```python
from build123d import *

# Parameters (mm, degrees)
SKIZZE1_R                       = 4.57
AUFSATZ_LINEAR_AUSTRAGEN1_DEPTH = 19
SCHNITT_LINEAR_AUSTRAGEN1_DEPTH = 20
VERRUNDUNG1_R                   = 0.5
KREISMUSTER1_COUNT              = 10
VERRUNDUNG1_OF_KREISMUSTER1_R   = 0.5
FASE1_SIZE                      = 0.2


with BuildPart() as part:
    # Skizze1 → Aufsatz-Linear austragen1 (new body)
    with BuildSketch(Plane(origin=(0, 0, 0), x_dir=(1, 0, 0), z_dir=(0, 1, 0))):
        Circle(SKIZZE1_R)
    extrude(amount=AUFSATZ_LINEAR_AUSTRAGEN1_DEPTH)

    # Skizze12 → Schnitt-Linear austragen1 (cut, through all)
    with BuildSketch(Plane(origin=(0, 19, 0), x_dir=(1, 0, 0), z_dir=(0, 1, 0))):
        with BuildLine():
            Line((-1.2, 4.409637173), (-0.808470756, 3.57))
            Line((-0.808470756, 3.57), (0.808470756, 3.57))
            Line((0.808470756, 3.57), (1.2, 4.409637173))
            ThreePointArc((1.2, 4.409637173), (0, 4.57), (-1.2, 4.409637173))
        make_face()
    schnitt_linear_austragen1 = extrude(amount=-SCHNITT_LINEAR_AUSTRAGEN1_DEPTH, mode=Mode.SUBTRACT)

    # Verrundung1
    verrundung1_edges = [part.edges().sort_by_distance(p)[0] for p in [
        (0.808470756, 9.5, -3.57),
        (-0.808470756, 9.5, -3.57),
    ]]
    fillet(verrundung1_edges, radius=VERRUNDUNG1_R)

    # Kreismuster1: Schnitt-Linear austragen1 ×10 about axis
    kreismuster1_axis = Axis((0, 0, 0), (0, 1, 0))
    for i in range(1, KREISMUSTER1_COUNT):
        add(schnitt_linear_austragen1.rotate(kreismuster1_axis, i * 360 / KREISMUSTER1_COUNT), mode=Mode.SUBTRACT)

    # Verrundung1 of Kreismuster1
    verrundung1_of_kreismuster1_edges = [part.edges().sort_by_distance(p)[0] for p in [
        (-1.44432677, 9.5, -3.363397857),
        (-2.752459932, 9.5, -2.412983483),
        (-3.14544056, 9.5, -1.872092051),
        (-3.645102966, 9.5, -0.334289289),
        (-3.645102966, 9.5, 0.334289289),
        (-3.14544056, 9.5, 1.872092051),
        (-2.752459932, 9.5, 2.412983483),
        (-1.44432677, 9.5, 3.363397857),
        (-0.808470756, 9.5, 3.57),
        (0.808470756, 9.5, 3.57),
        (1.44432677, 9.5, 3.363397857),
        (2.752459932, 9.5, 2.412983483),
        (3.14544056, 9.5, 1.872092051),
        (3.645102966, 9.5, 0.334289289),
        (3.645102966, 9.5, -0.334289289),
        (3.14544056, 9.5, -1.872092051),
        (2.752459932, 9.5, -2.412983483),
        (1.44432677, 9.5, -3.363397857),
    ]]
    fillet(verrundung1_of_kreismuster1_edges, radius=VERRUNDUNG1_OF_KREISMUSTER1_R)

    # Skizze13 → Schnitt-Rotation1 (revolve, cut)
    with BuildSketch(Plane(origin=(0, 0, 0), x_dir=(0, 0, -1), z_dir=(1, 0, 0))):
        Polygon((-1.995, 0), (-10.076763041, 0), (-10.076763041, 19), (-1.995, 19), (-1.995, 17), (-2.75, 17), (-2.75, 16.5), (-6.450923694, 16.5), (-6.450923694, 2.5), (-2.75, 2.5), (-2.75, 2), (-1.995, 2), align=None)
    revolve(axis=Axis((0, -5.607699778, 0), (0, 1, 0)), mode=Mode.SUBTRACT)

    # Fase1
    fase1_edges = [part.edges().sort_by_distance(p)[0] for p in [
        (0, 19, -1.995),
        (0, 0, -1.995),
        (0, 2, -2.75),
        (0, 17, -2.75),
    ]]
    chamfer(fase1_edges, length=FASE1_SIZE)

    # Skizze14 → Schnitt-Rotation2 (revolve, cut)
    with BuildSketch(Plane(origin=(0, 0, 0), x_dir=(0, 0, -1), z_dir=(1, 0, 0))):
        Polygon((0, 0), (-0.6, 0), (-0.6, 1.5), (0, 1.748528137), align=None)
    revolve(axis=Axis((0, -2.816169131, 0), (0, 1, 0)), mode=Mode.SUBTRACT)


solid = part.part
```
For this review, take the finished solid that the model builds, in its own axes (mm). A direction names the side the tool comes from. Round coordinates to 2 decimals unless told otherwise and drop trailing zeros.
Q1. Wall thickness on line 1 (X direction, y = 1.05, z = 0) (3 decimals); line 2 (Y direction, x = 0.25, z = -3); line 3 (X direction, y = 14.5, z = -3.5): over which ranges is each line inside the solid? List them lowest first.
Findings below:
line 1: x = -1.995 to -0.6, 0.6 to 1.995
line 2: y = 2.5 to 16.5
line 3: x = -1.5 to 1.5
Q2. Insertion check: P1, Ø0.8, axis at x = 0, y = 7.5, coming from the -Z side; P2, Ø4, axis at y = 13, z = 1, coming from the -X side; P3, Ø2, axis at x = -1, y = 8, coming from the +Z side; P4, Ø1.5, axis at y = 11.5, z = -1.5, coming from the +X side. Each pin has a flat end and moves straight along its axis. Give the tip position at first contact, or say it passes through.
Findings below:
P1: stops at z = -3.57
P2: stops at x = -4.57
P3: stops at z = 4.41
P4: stops at x = 3.55
Q3. Machinability: for faces 4 (the flat face through (3.397, 9.598, 1.097)), 5 (the cylindrical face through (-2.44, 2.35, 1.27)), 6 (the cylindrical face through (-1.05, 16.65, 2.54)), 7 (the flat face through (0, 10, 3.57)), which of the approach directions +Z, -Z, +X, -X, +Y, -Y give a long, thin tool a straight path to every point of the face, cutting with its end or side? Answer none if there is none.
Findings below:
face 4: +X, +Y, -Y
face 5: -Y
face 6: +Y
face 7: +Z, +Y, -Y
Q4. Mouldability with a two-part tool opening along Z and no side actions: class faces 1 (the flat face through (-1, 17, 2)), 2 (the flat face through (-3.397, 9.598, -1.097)), 3 (the flat face through (0, 10, -3.57)) as pulls with the +Z half, pulls with the -Z half, needs draft (parallel to the pull), parting line crosses it, or undercut.
Findings below:
face 1: needs draft
face 2: undercut
face 3: pulls with the -Z half
